from build123d import *

# Parameters (mm, degrees)
F0_W        = 57.5
F0_H        = 22
F0_W_2      = 55.5
F0_H_2      = 20
F1_DEPTH    = 9
F2_W        = 57.5
F2_H        = 22
F3_DEPTH    = 1
F5_DEPTH    = 1
F6_W        = 5.9
F6_H        = 6
F7_DEPTH    = 50
F8_R        = 1.6
F9_DEPTH    = 5.9
F10_W       = 1.5
F10_H       = 20
F11_DEPTH   = 2
F12_R       = 1
F13_R       = 1
F14_R       = 1.5
F15_DEPTH   = 1
F16_W       = 2.6
F16_H       = 1.2
F17_DEPTH   = 4
F18_SIZE2   = 0.5
F18_SIZE    = 1
F18_2_SIZE2 = 0.5
F18_2_SIZE  = 1
F19_SIZE2   = 1
F19_SIZE    = 0.5


with BuildPart() as f1:
    # F0 (on Top) → F1 (new body)
    with BuildSketch(Plane.XY):
        Rectangle(F0_W, F0_H)
        Rectangle(F0_W_2, F0_H_2, mode=Mode.SUBTRACT)
    extrude(amount=F1_DEPTH)

    # F2 (on Top) → F3 (join)
    with BuildSketch(Plane.XY):
        Rectangle(F2_W, F2_H)
    extrude(amount=F3_DEPTH)

    # F4 (on face) → F5 (cut, through all)
    with BuildSketch(Plane.XZ.offset(11)):
        with BuildLine():
            Line((2, 9), (-2, 9))
            Line((-2, 9), (-2, 5))
            ThreePointArc((-2, 5), (-1.7071067812, 4.2928932188), (-1, 4))
            Line((-1, 4), (1, 4))
            ThreePointArc((1, 4), (1.7071067812, 4.2928932188), (2, 5))
            Line((2, 5), (2, 9))
        make_face()
    extrude(amount=-F5_DEPTH, mode=Mode.SUBTRACT)

    # F6 (on face) → F7 (join)
    with BuildSketch(Plane.XZ.offset(11)):
        with Locations((17.75, 3)):
            Rectangle(F6_W, F6_H)
    extrude(amount=F7_DEPTH)

    # F8 (on face) → F9 (cut, through all)
    with BuildSketch(Plane.YZ.offset(20.7)):
        with Locations((-57, 3)):
            Circle(F8_R)
    extrude(amount=-F9_DEPTH, mode=Mode.SUBTRACT)

    # F10 (on face) → F11 (join)
    with BuildSketch(Plane.XY.offset(1)):
        with Locations((-25.5, 0)):
            Rectangle(F10_W, F10_H)
        with Locations((25.5, 0)):
            Rectangle(F10_W, F10_H)
    extrude(amount=F11_DEPTH)

    # F12
    f12_edges = [f1.edges().sort_by_distance(p)[0] for p in [
        (-28.75, -11, 4.5),
        (28.75, -11, 4.5),
        (28.75, 11, 4.5),
        (-28.75, 11, 4.5),
    ]]
    fillet(f12_edges, radius=F12_R)

    # F13
    f13_edges = [f1.edges().sort_by_distance(p)[0] for p in [
        (-27.75, 10, 5),
        (27.75, 10, 5),
        (27.75, -10, 5),
        (-27.75, -10, 5),
    ]]
    fillet(f13_edges, radius=F13_R)

    # F14 (on face) → F15 (cut, through all)
    with BuildSketch(Plane.YZ.offset(28.75)):
        with Locations((0, 6.5)):
            Circle(F14_R)
    extrude(amount=-F15_DEPTH, mode=Mode.SUBTRACT)

    # F16 (on face) → F17 (join)
    with BuildSketch(Plane.XY.offset(1)):
        with Locations((26.45, 2)):
            Rectangle(F16_W, F16_H)
        with Locations((-26.45, 2)):
            Rectangle(F16_W, F16_H)
    extrude(amount=F17_DEPTH)

    # F18
    f18_edges = [f1.edges().sort_by_distance(p)[0] for p in [
        (-25.15, 2.6, 4),
    ]]
    f18_side = f1.faces().sort_by_distance((-26.65122, 2.6, 3.268293))[0]
    chamfer(f18_edges, length=F18_SIZE, length2=F18_SIZE2, reference=f18_side)

    # F18#2
    f18_2_edges = [f1.edges().sort_by_distance(p)[0] for p in [
        (-25.15, 1.4, 4),
    ]]
    f18_2_side = f1.faces().sort_by_distance((-26.65122, 1.4, 3.268293))[0]
    chamfer(f18_2_edges, length=F18_2_SIZE, length2=F18_2_SIZE2, reference=f18_2_side)

    # F19
    f19_edges = [f1.edges().sort_by_distance(p)[0] for p in [
        (25.15, 2.6, 4),
        (25.15, 1.4, 4),
    ]]
    f19_side = f1.faces().sort_by_distance((25.15, 2, 4))[0]
    chamfer(f19_edges, length=F19_SIZE, length2=F19_SIZE2, reference=f19_side)


solid = f1.part
The listing builds one solid part. Answer for the finished solid, in the listing's coordinates (mm). A direction names the side the tool comes from. Coordinates: 2 decimals unless noted, no trailing zeros. Order: outer loops, then holes, each group sorted by start corner. A loop starts at its lowest first (then second) coordinate and runs counter-clockwise, first axis right, second up. Notation, with made-up numbers: (-22, 38.25) -> (22, 38.25) arc R14 ccw to (22, 60.25) -> close; hole circle Ø11 at (43.25, 73). An arc over 180 degrees is marked (long way). Answer in a Markdown table with one row per item. Add a question column.
Item 1: Find section C-C (x = 4). Write down the section's boundary in (y, z).
Item 2: Which of the six approach directions +Z, -Z, +X, -X, +Y, -Y give full straight-line access (tool end or side, diameter ignored) to faces 4 (the face through (20.7, -36, 3)), 5 (the face through (28, 0, 5)), 6 (the face through (-24.75, 0, 2)), 7 (the face through (0, 11, 4))?
Item 3: Determine the mould class of faces 1 (the face through (-8.7, 10.6, 9)), 2 (the face through (18, -61, 3)), 3 (the face through (27.75, 0, 4)) for opening direction Y: +Y half, -Y half, draft (parallel to the pull), parting line (faces both ways), or undercut.
Item 4: Each of these flat-tipped pins is pushed along its axis until it touches: P1, Ø1, axis at x = 26.5, y = 2, coming from the +Z side; P2, Ø1.2, axis at x = 25.5, y = -3.5, coming from the +Z side; P3, Ø10, axis at x = -15.5, y = -9, coming from the -Z side; P4, Ø4, axis at y = -44.5, z = 4.5, coming from the +X side. Where does it stop, or does it pass through?
Item 5: Find the intervals of material crossed by L1, parallel to Z at x = 19, y = -57; L2, parallel to X at y = -7, z = 4.5; L3, parallel to X at y = -4, z = 2.75, in increasing order. Write a range as from..to.
Item 6: Find section B-B (x = 16.5). Write down the section's boundary in (y, z), then the cut area to 3 significant figures.
Item 7: Find section D-D (y = 0). Write down the section's boundary in (x, z).
Item 8: Find section A-A (y = -57). Write down the section's boundary in (x, z).
Result set:
| question | item | result |
|---|---|---|
| 1 | outline | (-11, 0) -> (11, 0) -> (11, 9) -> (10, 9) -> (10, 1) -> (-10, 1) -> (-10, 9) -> (-11, 9) -> close |
| 2 | face 4 | +Z, -Z, +X, -Y |
| 2 | face 5 | +X |
| 2 | face 6 | +Z |
| 2 | face 7 | +Z, -Z, +X, -X, +Y |
| 3 | face 1 | draft |
| 3 | face 2 | -Y half |
| 3 | face 3 | undercut |
| 4 | P1 | stops at z = 5 |
| 4 | P2 | stops at z = 3 |
| 4 | P3 | stops at z = 0 |
| 4 | P4 | stops at x = 20.7 |
| 5 | L1 | z = 0..1.4, 4.6..6 |
| 5 | L2 | x = -28.75..-27.75, 27.75..28.75 |
| 5 | L3 | x = -28.75..-27.75, -26.25..-24.75, 24.75..26.25, 27.75..28.75 |
| 6 | outline | (-61, 0) -> (11, 0) -> (11, 9) -> (10, 9) -> (10, 1) -> (-10, 1) -> (-10, 9) -> (-11, 9) -> (-11, 6) -> (-61, 6) -> close; hole circle Ø3.2 at (-57, 3) |
| 6 | area | 330 mm² |
| 7 | outline | (-28.75, 0) -> (28.75, 0) -> (28.75, 5) -> (27.75, 5) -> (27.75, 1) -> (26.25, 1) -> (26.25, 3) -> (24.75, 3) -> (24.75, 1) -> (-24.75, 1) -> (-24.75, 3) -> (-26.25, 3) -> (-26.25, 1) -> (-27.75, 1) -> (-27.75, 9) -> (-28.75, 9) -> close; (27.75, 8) -> (28.75, 8) -> (28.75, 9) -> (27.75, 9) -> close |
| 8 | outline | (14.8, 0) -> (20.7, 0) -> (20.7, 1.4) -> (14.8, 1.4) -> close; (14.8, 4.6) -> (20.7, 4.6) -> (20.7, 6) -> (14.8, 6) -> close |
